Could you check a few things on this model? Use its own coordinates, in mm. A direction names the side the tool comes from. Round coordinates to 2 decimals unless told otherwise and drop trailing zeros. Order: outer loops, then holes, each group sorted by start corner. A loop starts at its lowest first (then second) coordinate and runs counter-clockwise, first axis right, second up. Notation, with made-up numbers: (-1, 2.5) -> (24, 2.5) arc R21 ccw to (24, 23.5) -> close; hole circle Ø9 at (85, 86). An arc over 180 degrees is marked (long way). One line per question, with ' | ' between items.
```python
from build123d import *

# Parameters (mm, degrees)
SKETCH1_W           = 381
SKETCH1_H           = 152.4
BOSS_EXTRUDE2_DEPTH = 12.7
SKETCH2_W           = 127
SKETCH2_H           = 127
CUT_EXTRUDE1_DEPTH  = 12.7
SKETCH3_W           = 19.05
SKETCH3_H           = 19.05
SKETCH3_W_2         = 76.2
SKETCH3_H_2         = 57.15
CUT_EXTRUDE2_DEPTH  = 12.7
SKETCH4_W           = 4.233333334
SKETCH4_H           = 127
BOSS_EXTRUDE3_DEPTH = 114.3


with BuildPart() as part:
    # Sketch1 → Boss-Extrude2 (new body)
    with BuildSketch(Plane(origin=(0, 0, 0), x_dir=(0, 0, -1), z_dir=(1, 0, 0))):
        with Locations((-190.5, 76.2)):
            Rectangle(SKETCH1_W, SKETCH1_H)
    extrude(amount=BOSS_EXTRUDE2_DEPTH)

    # Sketch2 → Cut-Extrude1 (cut)
    with BuildSketch(Plane(origin=(12.7, 0, 0), x_dir=(0, 0, -1), z_dir=(1, 0, 0))):
        with Locations((-190.5, 88.9)):
            Rectangle(SKETCH2_W, SKETCH2_H)
    extrude(amount=-CUT_EXTRUDE1_DEPTH, mode=Mode.SUBTRACT)

    # Sketch3 → Cut-Extrude2 (cut)
    with BuildSketch(Plane(origin=(12.7, 0, 0), x_dir=(0, 0, -1), z_dir=(1, 0, 0))):
        with Locations((-100.0125, 92.075)):
            Rectangle(SKETCH3_W, SKETCH3_H)
        with Locations((-63.5, 92.075)):
            Rectangle(SKETCH3_W, SKETCH3_H)
        with Locations((-26.9875, 92.075)):
            Rectangle(SKETCH3_W, SKETCH3_H)
        with Locations((-100.0125, 53.340985209)):
            Rectangle(SKETCH3_W, SKETCH3_H)
        with Locations((-63.5, 53.340985209)):
            Rectangle(SKETCH3_W, SKETCH3_H)
        with Locations((-26.9875, 53.340985209)):
            Rectangle(SKETCH3_W, SKETCH3_H)
        with Locations((-317.5, 60.325)):
            Rectangle(SKETCH3_W_2, SKETCH3_H_2)
    extrude(amount=-CUT_EXTRUDE2_DEPTH, mode=Mode.SUBTRACT)

    # Sketch4 → Boss-Extrude3 (add)
    with BuildSketch(Plane(origin=(0, 25.4, 0), x_dir=(1, 0, 0), z_dir=(0, 1, 0))):
        with Locations((6.35, -190.5)):
            Rectangle(SKETCH4_W, SKETCH4_H)
    extrude(amount=BOSS_EXTRUDE3_DEPTH)


solid = part.part
```
1. I want a section at C-C on y = 109.5. List the corners of the cut face in (x, z) for me, and give its area (3 significant figures).
From the geometry:
outline: (0, 0) -> (12.7, 0) -> (12.7, 127) -> (8.47, 127) -> (8.47, 254) -> (12.7, 254) -> (12.7, 381) -> (0, 381) -> (0, 254) -> (4.23, 254) -> (4.23, 127) -> (0, 127) -> close | area: 3,760 mm²
2. I need wall thicknesses on probe 1 along Z at (x, y) = (11.5, 51.5) (1 decimal); probe 2 along Z at (x, y) = (11.25, 90) (1 decimal); probe 3 along Z at (x, y) = (1.25, 66). Which ranges of each line are inside material? Lowest first, please.
From the geometry:
probe 1: z = 0 to 17.5, 36.5 to 54, 73 to 90.5, 109.5 to 127, 254 to 279.4, 355.6 to 381 | probe 2: z = 0 to 17.5, 36.5 to 54, 73 to 90.5, 109.5 to 127, 254 to 381 | probe 3: z = 0 to 127, 254 to 279.4, 355.6 to 381
3. I want a section at A-A on y = 57.5. List the corners of the cut face in (x, z) for me (1 decimal), and give its area (3 significant figures).
From the geometry:
outline: (0, 0) -> (12.7, 0) -> (12.7, 17.5) -> (0, 17.5) -> close; (0, 36.5) -> (12.7, 36.5) -> (12.7, 54) -> (0, 54) -> close; (0, 73) -> (12.7, 73) -> (12.7, 90.5) -> (0, 90.5) -> close; (0, 109.5) -> (12.7, 109.5) -> (12.7, 127) -> (8.5, 127) -> (8.5, 254) -> (12.7, 254) -> (12.7, 279.4) -> (0, 279.4) -> (0, 254) -> (4.2, 254) -> (4.2, 127) -> (0, 127) -> close; (0, 355.6) -> (12.7, 355.6) -> (12.7, 381) -> (0, 381) -> close | area: 2,070 mm²
4. I want a section at D-D on z = 241. List the corners of the cut face in (x, y) for me, and give its area (3 significant figures).
From the geometry:
outline: (0, 0) -> (12.7, 0) -> (12.7, 25.4) -> (8.47, 25.4) -> (8.47, 139.7) -> (4.23, 139.7) -> (4.23, 25.4) -> (0, 25.4) -> close | area: 806 mm²
5. If we mould it in two halves opening along Z, with no side actions, what happens to faces 4 (the face through (0, 10, 193)), 5 (the face through (6, 53, 90.488))? For each: pulls with the +Z half, pulls with the -Z half, needs draft (parallel to the pull), parting line crosses it, or undercut.
From the geometry:
face 4: needs draft | face 5: undercut
6. I'm going to push flat-ended pins straight in: pin 1 (6 mm diameter, centred on x = 10.5, y = 49, fed in from -Z); pin 2 (3.5 mm diameter, centred on x = 1, z = 169, fed in from +Y); pin 3 (10 mm diameter, centred on y = 63, z = 248, fed in from -X); pin 4 (1.5 mm diameter, centred on y = 116.5, z = 189.5, fed in from +X). Where does each tip first touch, or does it pass through?
From the geometry:
pin 1: stops at z = 0 | pin 2: stops at y = 25.4 | pin 3: stops at x = 4.23 | pin 4: stops at x = 8.47
7. I want a section at B-B on z = 289.5. List the corners of the cut face in (x, y) for me, and give its area (3 significant figures).
From the geometry:
outline: (0, 0) -> (12.7, 0) -> (12.7, 31.75) -> (0, 31.75) -> close; (0, 88.9) -> (12.7, 88.9) -> (12.7, 152.4) -> (0, 152.4) -> close | area: 1,210 mm²
8. On a 3-axis mill with a long thin cutter (end or side, diameter ignored), from which of +Z, -Z, +X, -X, +Y, -Y can I reach the whole of each face in a straight line? I mean faces 1 (the face through (4, 88, 254)), 2 (the face through (6, 62.866, 100)), 3 (the face through (8.467, 82, 191)). Say none if no direction works.
From the geometry:
face 1: +Y | face 2: +X, -X | face 3: +X, +Y
